Design review of the part shown in the three views and the two pictorial views. Dimensions are in mm from the part's minimum x, y and z. A direction names the side the tool comes from. Round coordinates to 2 decimals unless told otherwise and drop trailing zeros. Write each loop counter-clockwise with the first axis right and the second up, starting at its lowest first coordinate (ties: lowest second). Pieces come first, ordered by that corner, then holes. Notation, with made-up numbers: (65.5, 5) - (75.5, 5) arc R17 cw to (75.5, 12) - close; hole circle Ø5 at (44, 57.5). An arc over 180 degrees is marked (long way). One line per item, written item: value. Start each with the question number.
Q1. Clearance check with flat-ended pins moving along their axes: pin 1 Ø3.5 at (x, z) = (54.5, 36.1) entering from +Y; pin 2 Ø2 at (y, z) = (9.5, 23.5) entering from +X; pin 3 Ø4 at (y, z) = (9, 30.5) entering from -X. State where each tip first meets the part, or that it passes through.
Q2. Add section C-C on z = 21. Write out the cut boundary in (x, y), and give its area (3 significant figures).
Q3. Add section D-D on y = 9. Write out the cut boundary in (x, z).
Q4. For probe 1 along X at (y, z) = (2.55, 36.1); probe 2 along X at (y, z) = (6, 38), list the stretches that pass through material, from the lowest coordinate up.
Q5. Add section B-B on z = 10. Write out the cut boundary in (x, y), and give its area (3 significant figures).
Q6. Add section A-A on x = 5. Write out the cut boundary in (y, z).
Q7. Tool access review of the marked faces 1, 2 and 3: name each direction out of +Z, -Z, +X, -X, +Y, -Y from which nothing blocks a thin tool from reaching the whole face with its end or side.
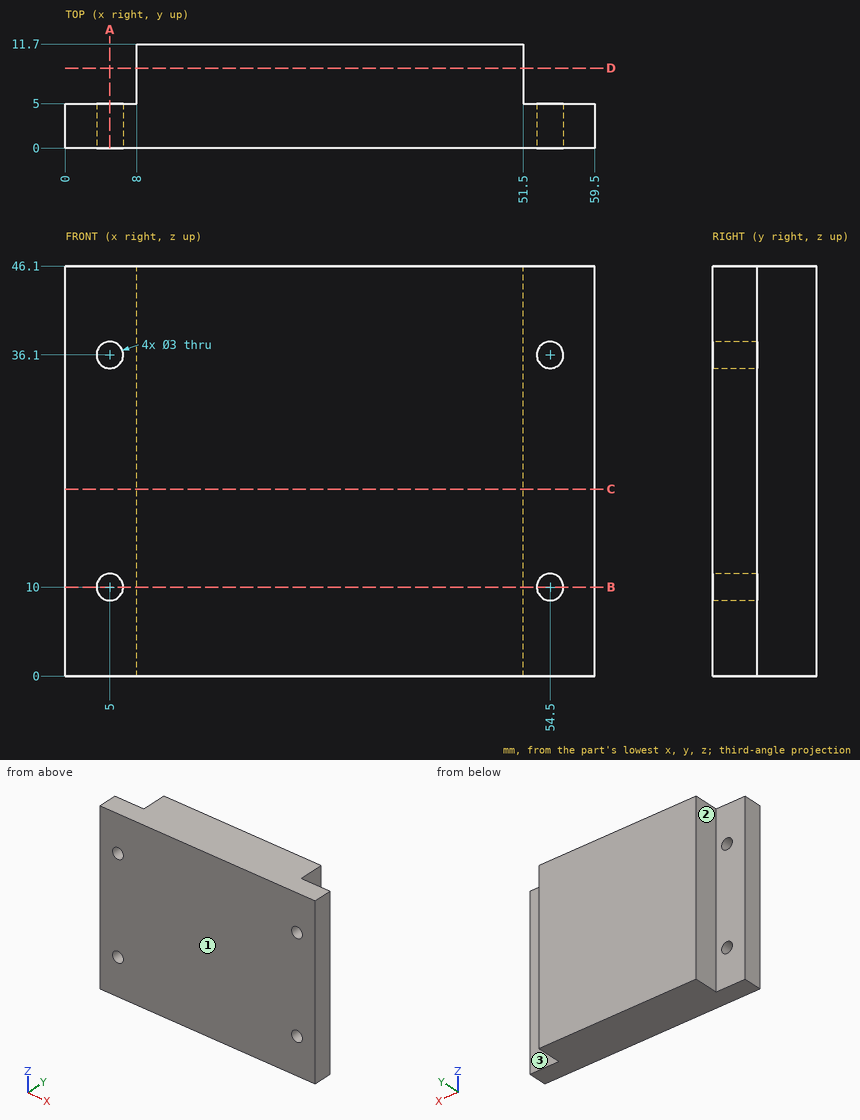
Result set:
1. pin 1: stops at y = 5
1. pin 2: stops at x = 51.5
1. pin 3: stops at x = 8
2. outline: (0, 0) - (59.5, 0) - (59.5, 5) - (51.5, 5) - (51.5, 11.7) - (8, 11.7) - (8, 5) - (0, 5) - close
2. area: 589 mm^2
3. outline: (8, 0) - (51.5, 0) - (51.5, 46.1) - (8, 46.1) - close
4. probe 1: x = 0 to 3.5, 6.5 to 53, 56 to 59.5
4. probe 2: x = 8 to 51.5
5. outline: (0, 0) - (3.5, 0) - (3.5, 5) - (0, 5) - close; (6.5, 0) - (53, 0) - (53, 5) - (51.5, 5) - (51.5, 11.7) - (8, 11.7) - (8, 5) - (6.5, 5) - close; (56, 0) - (59.5, 0) - (59.5, 5) - (56, 5) - close
5. area: 559 mm^2
6. outline: (0, 0) - (5, 0) - (5, 8.5) - (0, 8.5) - close; (0, 11.5) - (5, 11.5) - (5, 34.6) - (0, 34.6) - close; (0, 37.6) - (5, 37.6) - (5, 46.1) - (0, 46.1) - close
7. face 1: +Z, -Z, +X, -X, -Y
7. face 2: +Z, -Z, -X, +Y
7. face 3: +Z, -Z, +X, +Y
